```python
from build123d import *

# Parameters (mm, degrees)
SKETCH1_W             = 40.5
SKETCH1_H             = 0.76
SKETCH2_R             = 1.6
CUT_EXTRUDE1_DEPTH    = 155.151151796
CIRPATTERN1_START     = 6.175
CIRPATTERN1_OUTLINE_R = 1.6
CIRPATTERN1_DEPTH     = 0.76
SKETCH4_R             = 1.6
CUT_EXTRUDE3_DEPTH    = 155.151151796


# Read off the part's stored shape, not the designer's step: CirPattern1
with BuildPart() as part:
    # Sketch1 → Revolve1 (revolve)
    with BuildSketch(Plane.XY, mode=Mode.PRIVATE) as revolve1_sk:
        with Locations((-88.75, 6.555)):
            Rectangle(SKETCH1_W, SKETCH1_H)
    revolve(revolve1_sk.sketch.rotate(Axis((0, -200069.047495165, 0), (0, 1, 0)), 270), axis=Axis((0, -200069.047495165, 0), (0, 1, 0)))

    # Sketch2 → Cut-Extrude1 (cut, through all)
    with BuildSketch(Plane(origin=(0, 6.935, 0), x_dir=(1, 0, 0), z_dir=(0, 1, 0))):
        with Locations(Location((0, 72, 0), (0, 0, 270))):
            Circle(SKETCH2_R)
    extrude(amount=-CUT_EXTRUDE1_DEPTH, mode=Mode.SUBTRACT)

    # CirPattern1 outline → CirPattern1 (cut)
    with BuildSketch(Plane(origin=(0, 0, 0), x_dir=(1, 0, 0), z_dir=(0, 1, 0)).offset(CIRPATTERN1_START)):
        with Locations((18.634971247, 69.546659493)):
            Circle(CIRPATTERN1_OUTLINE_R)
        with Locations((-18.634971247, 69.546659493)):
            Circle(CIRPATTERN1_OUTLINE_R)
        with Locations((-36, 62.353829072)):
            Circle(CIRPATTERN1_OUTLINE_R)
        with Locations((-50.911688245, 50.911688245)):
            Circle(CIRPATTERN1_OUTLINE_R)
        with Locations((-62.353829072, 36)):
            Circle(CIRPATTERN1_OUTLINE_R)
        with Locations((-69.546659493, 18.634971247)):
            Circle(CIRPATTERN1_OUTLINE_R)
        with Locations((-72, 0)):
            Circle(CIRPATTERN1_OUTLINE_R)
        with Locations((36, 62.353829072)):
            Circle(CIRPATTERN1_OUTLINE_R)
        with Locations((50.911688245, 50.911688245)):
            Circle(CIRPATTERN1_OUTLINE_R)
        with Locations((62.353829072, 36)):
            Circle(CIRPATTERN1_OUTLINE_R)
        with Locations((69.546659493, 18.634971247)):
            Circle(CIRPATTERN1_OUTLINE_R)
        with Locations((72, 0)):
            Circle(CIRPATTERN1_OUTLINE_R)
        with Locations((69.546659493, -18.634971247)):
            Circle(CIRPATTERN1_OUTLINE_R)
        with Locations((62.353829072, -36)):
            Circle(CIRPATTERN1_OUTLINE_R)
        with Locations((50.911688245, -50.911688245)):
            Circle(CIRPATTERN1_OUTLINE_R)
        with Locations((36, -62.353829072)):
            Circle(CIRPATTERN1_OUTLINE_R)
        with Locations((18.634971247, -69.546659493)):
            Circle(CIRPATTERN1_OUTLINE_R)
        with Locations((0, -72)):
            Circle(CIRPATTERN1_OUTLINE_R)
        with Locations((-18.634971247, -69.546659493)):
            Circle(CIRPATTERN1_OUTLINE_R)
        with Locations((-36, -62.353829072)):
            Circle(CIRPATTERN1_OUTLINE_R)
        with Locations((-50.911688245, -50.911688245)):
            Circle(CIRPATTERN1_OUTLINE_R)
        with Locations((-62.353829072, -36)):
            Circle(CIRPATTERN1_OUTLINE_R)
        with Locations((-69.546659493, -18.634971247)):
            Circle(CIRPATTERN1_OUTLINE_R)
    extrude(amount=CIRPATTERN1_DEPTH, mode=Mode.SUBTRACT)

    # Sketch4 → Cut-Extrude3 (cut, through all)
    with BuildSketch(Plane(origin=(0, 6.935, 0), x_dir=(1, 0, 0), z_dir=(0, 1, 0))):
        with Locations(Location((-103.194571877, -21.934683381, 0), (0, 0, 270))):
            Circle(SKETCH4_R)
        with Locations(Location((-105.407458575, -4.417881468, 0), (0, 0, 270))):
            Circle(SKETCH4_R)
        with Locations(Location((-104.668100989, -13.222656141, 0), (0, 0, 270))):
            Circle(SKETCH4_R)
        with Locations(Location((-100.336462469, 32.601292907, 0), (0, 0, 270))):
            Circle(SKETCH4_R)
        with Locations(Location((104.295371407, 15.897342642, 0), (0, 0, 270))):
            Circle(SKETCH4_R)
        with Locations(Location((100.708995202, 31.43164465, 0), (0, 0, 270))):
            Circle(SKETCH4_R)
        with Locations(Location((94.822771885, 46.248155986, 0), (0, 0, 270))):
            Circle(SKETCH4_R)
        with Locations(Location((-103.194571877, 21.934683381, 0), (0, 0, 270))):
            Circle(SKETCH4_R)
        with Locations(Location((-104.668100989, 13.222656141, 0), (0, 0, 270))):
            Circle(SKETCH4_R)
        with Locations(Location((-105.407458575, 4.417881468, 0), (0, 0, 270))):
            Circle(SKETCH4_R)
        with Locations(Location((89.469074145, -55.906482377, 0), (0, 0, 270))):
            Circle(SKETCH4_R)
        with Locations(Location((-44.130594647, 95.826617472, 0), (0, 0, 270))):
            Circle(SKETCH4_R)
        with Locations(Location((-62.82106423, 84.757087545, 0), (0, 0, 270))):
            Circle(SKETCH4_R)
        with Locations(Location((-78.848228037, 70.094271773, 0), (0, 0, 270))):
            Circle(SKETCH4_R)
        with Locations(Location((-91.532612735, 52.45980181, 0), (0, 0, 270))):
            Circle(SKETCH4_R)
        with Locations(Location((94.822771885, -46.248155986, 0), (0, 0, 270))):
            Circle(SKETCH4_R)
        with Locations(Location((100.708995202, -31.43164465, 0), (0, 0, 270))):
            Circle(SKETCH4_R)
        with Locations(Location((104.295371407, -15.897342642, 0), (0, 0, 270))):
            Circle(SKETCH4_R)
        with Locations(Location((105.5, 0, 0), (0, 0, 270))):
            Circle(SKETCH4_R)
        with Locations(Location((76.122528254, -73.04526468, 0), (0, 0, 270))):
            Circle(SKETCH4_R)
        with Locations(Location((89.469074145, 55.906482377, 0), (0, 0, 270))):
            Circle(SKETCH4_R)
        with Locations(Location((76.122528254, 73.04526468, 0), (0, 0, 270))):
            Circle(SKETCH4_R)
        with Locations(Location((59.54875959, 87.08728513, 0), (0, 0, 270))):
            Circle(SKETCH4_R)
        with Locations(Location((40.450414858, 97.437230758, 0), (0, 0, 270))):
            Circle(SKETCH4_R)
        with Locations(Location((19.637170436, 103.656314507, 0), (0, 0, 270))):
            Circle(SKETCH4_R)
        with Locations(Location((-2.008593938, 105.480877653, 0), (0, 0, 270))):
            Circle(SKETCH4_R)
        with Locations(Location((-23.569203757, 102.833567643, 0), (0, 0, 270))):
            Circle(SKETCH4_R)
        with Locations(Location((-91.532612735, -52.45980181, 0), (0, 0, 270))):
            Circle(SKETCH4_R)
        with Locations(Location((-62.82106423, -84.757087545, 0), (0, 0, 270))):
            Circle(SKETCH4_R)
        with Locations(Location((-44.130594647, -95.826617472, 0), (0, 0, 270))):
            Circle(SKETCH4_R)
        with Locations(Location((-23.569203757, -102.833567643, 0), (0, 0, 270))):
            Circle(SKETCH4_R)
        with Locations(Location((-2.008593938, -105.480877653, 0), (0, 0, 270))):
            Circle(SKETCH4_R)
        with Locations(Location((19.637170436, -103.656314507, 0), (0, 0, 270))):
            Circle(SKETCH4_R)
        with Locations(Location((40.450414858, -97.437230758, 0), (0, 0, 270))):
            Circle(SKETCH4_R)
        with Locations(Location((59.54875959, -87.08728513, 0), (0, 0, 270))):
            Circle(SKETCH4_R)
        with Locations(Location((-78.848228037, -70.094271773, 0), (0, 0, 270))):
            Circle(SKETCH4_R)
        with Locations(Location((-100.336462469, -32.601292907, 0), (0, 0, 270))):
            Circle(SKETCH4_R)
    extrude(amount=-CUT_EXTRUDE3_DEPTH, mode=Mode.SUBTRACT)


solid = part.part
```
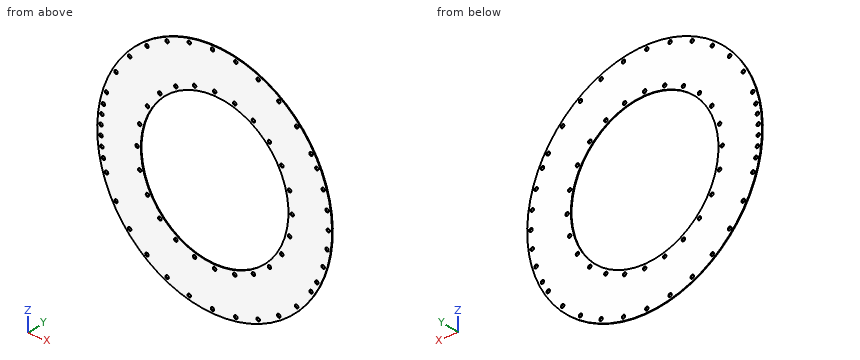
Read the model definition and answer for the solid it produces. Units are mm, in the model's axes. Give positions to 0.01 mm unless a question says otherwise; leave off trailing zeros. Write each loop counter-clockwise with the first axis right and the second up, starting at its lowest first coordinate (ties: lowest second). Pieces come first, ordered by that corner, then holes. Notation, with made-up numbers: M 44.5,-4 L 84.5,-4 A27 ccw 84.5,31 Z; hole C -4,26.5 d7. An arc over 180 degrees is marked long. Put each result on its own line as item: value. Start each with the question number.
1. Consider line 1 along X through (y, z) = (6.75, 0); line 2 along X through (y, z) = (6.6, 70); line 3 along X through (y, z) = (6.8, -36). Determine where each line is inside the solid, lowest interval first.
2. The part is cut by section B-B, the plane y = 6.55. Give the number of separate pieces and of enclosed holes in the cut face, and give its area (3 significant figures).
3. The part is cut by section A-A, the plane x = 10. Give the vertices of the cut face in (y, z) (3 decimals).
Final values:
1. line 1: x = -109 to -73.6, -70.4 to -68.5, 68.5 to 70.4, 73.6 to 103.9, 107.1 to 109
1. line 2: x = -83.55 to -80.45, -77.25 to -20.17, -17.1 to 17.1, 20.17 to 83.55
1. line 3: x = -102.88 to -63.95, -60.75 to -58.28, 58.28 to 60.75, 63.95 to 102.88
2. separate pieces: 1
2. enclosed holes: 62
2. area: 22,100 mm²
3. outline: M 6.175,-108.54 L 6.935,-108.54 L 6.935,-67.766 L 6.175,-67.766 Z; M 6.175,67.766 L 6.935,67.766 L 6.935,108.54 L 6.175,108.54 Z
